Here's how the part is built. I have some questions about the finished solid (model axes, mm). Face numbers are marked on the shaded views. A direction names the side the tool comes from. Coordinates: 2 decimals unless noted, no trailing zeros. Loops run counter-clockwise (first coordinate to the right, second up) from the corner with the lowest first, then second, coordinate; pieces in that order, holes last. Notation, with made-up numbers: (-6, 38.25) -> (45, 38.25) arc R16 cw to (45, 67.25) -> close; hole circle Ø1 at (-8.75, 15.5). An arc over 180 degrees is marked (long way). Answer as a JSON object with one key per item and string values. Group by question number.
1) I need wall thicknesses on probe 1 along X at (y, z) = (14.5, 7); probe 2 along Y at (x, z) = (65, 5.5); probe 3 along Z at (x, y) = (110, -6.5). Which ranges of each line are inside material? Lowest first, please. Write a range as [from, to].
2) Which directions (+Z, -Z, +X, -X, +Y, -Y) give clear straight access to the entire face, cutting with the end or side of a thin tool? Please do the marked faces 1 and 2.
3) I want a section at C-C (x = 25). Write out the boundary of the cut face in (y, z).
4) I want a section at A-A (y = -5). Write out the boundary of the cut face in (x, z), then the cut area to 3 significant figures.
5) I want a section at D-D (z = -24.5). Write out the boundary of the cut face in (x, y).
6) I want a section at B-B (z = 2). Write out the boundary of the cut face in (x, y).
7) I'm going to push a flat-ended pin straight in: pin 1 (18 mm diameter, centred on x = 97, z = -3.5, fed in from +Y). Where does the tip first touch, or does it pass through?
```python
from build123d import *

# Parameters (mm, degrees)
SKETCH1_W           = 60
SKETCH1_H           = 20
BOSS_EXTRUDE1_DEPTH = 130
SKETCH2_W           = 60
SKETCH2_H           = 60
BOSS_EXTRUDE2_DEPTH = 15
SKETCH3_R           = 4.767204383
CUT_EXTRUDE1_DEPTH  = 200


with BuildPart() as part:
    # Sketch1 → Boss-Extrude1 (new body)
    with BuildSketch(Plane(origin=(0, 0, 0), x_dir=(0, 0, -1), z_dir=(1, 0, 0))):
        with Locations((1.866028708, -8.133971292)):
            Rectangle(SKETCH1_W, SKETCH1_H)
    extrude(amount=BOSS_EXTRUDE1_DEPTH)

    # Sketch2 → Boss-Extrude2 (add)
    with BuildSketch(Plane(origin=(0, 1.866028708, 0), x_dir=(1, 0, 0), z_dir=(0, 1, 0))):
        with Locations((30, 1.866028708)):
            Rectangle(SKETCH2_W, SKETCH2_H)
    extrude(amount=BOSS_EXTRUDE2_DEPTH)

    # Sketch3 → Cut-Extrude1 (cut)
    with BuildSketch(Plane(origin=(130, 0, 0), x_dir=(0, 0, -1), z_dir=(1, 0, 0))):
        with Locations((0.210093723, -3.611871182)):
            Circle(SKETCH3_R)
    extrude(amount=-CUT_EXTRUDE1_DEPTH, mode=Mode.SUBTRACT)


solid = part.part
```
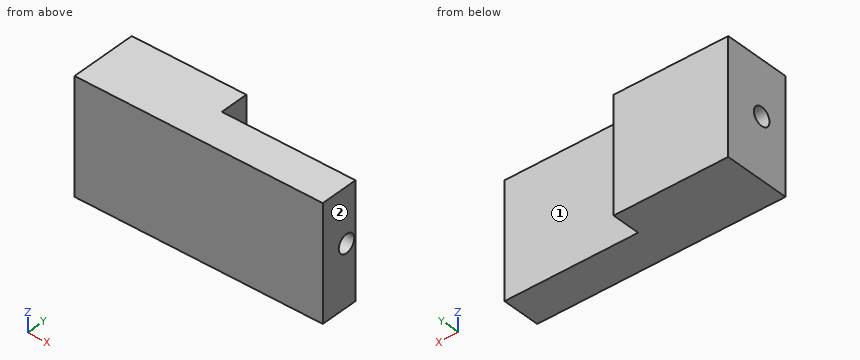
Determined:
{
 "1": {"probe 1": "[0, 60]", "probe 2": "[-18.13, 1.87]", "probe 3": "[-31.87, -4], [3.58, 28.13]"},
 "2": {"face 1": "+Z, -Z, +X, +Y", "face 2": "+Z, -Z, +X, +Y, -Y"},
 "3": {"outline": "(-18.13, -31.87) -> (16.87, -31.87) -> (16.87, 28.13) -> (-18.13, 28.13) -> close; hole circle Ø9.53 at (-3.61, -0.21)"},
 "4": {"outline": "(0, -31.87) -> (130, -31.87) -> (130, -4.77) -> (0, -4.77) -> close; (0, 4.35) -> (130, 4.35) -> (130, 28.13) -> (0, 28.13) -> close", "area": "6,610 mm^2"},
 "5": {"outline": "(0, -18.13) -> (130, -18.13) -> (130, 1.87) -> (60, 1.87) -> (60, 16.87) -> (0, 16.87) -> close"},
 "6": {"outline": "(0, -18.13) -> (130, -18.13) -> (130, -7.84) -> (0, -7.84) -> close; (0, 0.61) -> (130, 0.61) -> (130, 1.87) -> (60, 1.87) -> (60, 16.87) -> (0, 16.87) -> close"},
 "7": {"pin 1": "y = 1.87"}
}
